Design review of the part built by this model. Coordinates are the model's own, in mm. Round coordinates to 2 decimals unless told otherwise and drop trailing zeros. Order: outer loops, then holes, each group sorted by start corner. A loop starts at its lowest first (then second) coordinate and runs counter-clockwise, first axis right, second up. Notation, with made-up numbers: M 47,56 L 66,56 A27 ccw 66,78 Z; hole C 64,11 d1. An arc over 180 degrees is marked long. Write each question's results on one line, items separated by ' | '. Start each with the question number.
Item 1: Clearance check with flat-ended pins moving along their axes: pin 1 (4 mm diameter, centred on y = -4.5, z = -6, fed in from +X); pin 2 (1 mm diameter, centred on y = -2, z = -11.5, fed in from +X); pin 3 (4 mm diameter, centred on x = -6.5, y = -6.5, fed in from +Z). State where each tip first meets the part, or that it passes through.
Item 2: Take a section at B-B, the plane y = -1.5. Write out the cut boundary in (x, z) (3 decimals), plus the area to 3 significant figures.
Item 3: Take a section at A-A, the plane y = -8.5. Write out the cut boundary in (x, z) (3 decimals), plus the area to 3 significant figures.
Item 4: Wall thickness on line 1 (X direction, y = -3.5, z = -2.5); line 2 (X direction, y = -9, z = 1); line 3 (Z direction, x = 1, y = -8.5): over which ranges is each line inside the solid? List them lowest first. Write a range as [from, to].
```python
from build123d import *

# Parameters (mm, degrees)
F1_DEPTH = 9.525
F2_R     = 3.81


with BuildPart() as f1:
    # F0 (on Front) → F1 (new body)
    with BuildSketch(Plane.XZ):
        with BuildLine():
            ThreePointArc((15.875, 0), (0, 15.875), (-15.875, 0))
            ThreePointArc((-15.875, 0), (0, -15.875), (15.875, 0))
        make_face()
        with BuildLine():
            ThreePointArc((0, -3.175), (-2.2450640303, -2.2450640303), (-3.175, 0))
            ThreePointArc((-3.175, 0), (0, 3.175), (3.175, 0))
            ThreePointArc((3.175, 0), (2.2450640303, -2.2450640303), (0, -3.175))
        make_face(mode=Mode.SUBTRACT)
    extrude(amount=F1_DEPTH)

    # F2
    f2_edges = [f1.edges().sort_by_distance(p)[0] for p in [
        (15.875, -9.525, 0),
        (15.875, 0, 0),
    ]]
    fillet(f2_edges, radius=F2_R)


solid = f1.part
```
Results list:
1) pin 1: x = 15.36 | pin 2: x = 10.91 | pin 3: z = 15.19
2) outline: C 0,0 d30.19; hole C 0,0 d6.35 | area: 684 mm²
3) outline: C 0,0 d29.33; hole C 0,0 d6.35 | area: 644 mm²
4) line 1: [-15.66, -1.96], [1.96, 15.66] | line 2: [-13.96, -3.01], [3.01, 13.96] | line 3: [-14.63, -3.01], [3.01, 14.63]
